```python
from build123d import *

# Parameters (mm, degrees)
SKETCH1_R               = 9.398
BOSS_EXTRUDE1_DEPTH     = 24.892
SKETCH2_R               = 2.54
CUT_EXTRUDE1_DEPTH      = 1
CUT_EXTRUDE1_DEPTH_BACK = 25.892
SKETCH3_R               = 3.9878
CUT_EXTRUDE2_DEPTH      = 12.446


with BuildPart() as part:
    # Sketch1 → Boss-Extrude1 (new body)
    with BuildSketch(Plane.XY):
        Circle(SKETCH1_R)
    extrude(amount=BOSS_EXTRUDE1_DEPTH)

    # Sketch2 → Cut-Extrude1 (cut, two sides)
    with BuildSketch(Plane(origin=(0, 0, 0), x_dir=(-1, 0, 0), z_dir=(0, 0, -1))) as cut_extrude1_sk:
        Circle(SKETCH2_R)
    extrude(amount=CUT_EXTRUDE1_DEPTH, mode=Mode.SUBTRACT)
    extrude(cut_extrude1_sk.sketch, amount=-CUT_EXTRUDE1_DEPTH_BACK, mode=Mode.SUBTRACT)

    # Sketch3 → Cut-Extrude2 (cut)
    with BuildSketch(Plane(origin=(0, 0, 0), x_dir=(-1, 0, 0), z_dir=(0, 0, -1))):
        Circle(SKETCH3_R)
    extrude(amount=-CUT_EXTRUDE2_DEPTH, mode=Mode.SUBTRACT)


solid = part.part
```
Check sheet for the modelled part. Datum: model origin and axes. Units: mm. A direction names the side the tool comes from. Coordinates: 2 decimals unless noted, no trailing zeros. Order: outer loops, then holes, each group sorted by start corner. A loop starts at its lowest first (then second) coordinate and runs counter-clockwise, first axis right, second up. Notation, with made-up numbers: M 22,52 L 70,52 A33 cw 70,81 Z; hole C 3,22 d11. An arc over 180 degrees is marked long. One line per question, with ' | ' between items. Start each with the question number.
Item 1: Sectioned sample at B-B on y = 1. Record the cut outline in (x, z), and give its area (3 significant figures).
Item 2: Sectioned sample at C-C on z = 17. Record the cut outline in (x, y).
Item 3: Gauge pin test, flat ends, axial feed: P1, Ø2, axis at y = -7.5, z = 16, coming from the +X side; P2, Ø5, axis at x = 0.5, y = -2, coming from the -Z side; P3, Ø8, axis at x = -5, z = 9.5, coming from the +Y side. Record the tip position at first contact, or that the pin passes through.
Item 4: Access from +Z, -Z, +X, -X, +Y, -Y to the whole of each face (thin tool, end or side, straight path). Record for faces 5 (the cylindrical face through (-3.804, 1.198, 6.136)), 6 (the flat face through (2, -2, 24.892)).
Item 5: Mould release check, pull along X, two halves, no side actions. Record for faces 1 (the cylindrical face through (0.33, 2.52, 18.58)), 2 (the flat face through (4, -2, 0)), 3 (the cylindrical face through (-1.22, 9.32, 12.27)), 4 (the flat face through (0, -3, 12.446)): pulls with the +X half, pulls with the -X half, needs draft (parallel to the pull), parting line crosses it, or undercut.
Item 6: Material ranges on line 1 (Y direction, x = 0, z = 9.5); line 2 (Z direction, x = 2, y = -2.75); line 3 (X direction, y = 1.5, z = 11.75), recorded low to high.
Item 7: Sectioned sample at D-D on x = 4.5. Record the cut outline in (y, z).
Item 8: Sectioned sample at A-A on x = 0. Record the cut outline in (y, z).
Answer below:
1) outline: M -9.34,0 L -3.86,0 L -3.86,12.45 L -2.33,12.45 L -2.33,24.89 L -9.34,24.89 Z; M 2.33,12.45 L 3.86,12.45 L 3.86,0 L 9.34,0 L 9.34,24.89 L 2.33,24.89 Z | area: 311 mm^2
2) outline: C 0,0 d18.8; hole C 0,0 d5.08
3) P1: stops at x = 6.79 | P2: stops at z = 0 | P3: stops at y = 9.34
4) face 5: -Z | face 6: +Z, +X, -X, +Y, -Y
5) face 1: undercut | face 2: needs draft | face 3: parting line crosses it | face 4: undercut
6) line 1: y = -9.4 to -3.99, 3.99 to 9.4 | line 2: z = 12.45 to 24.89 | line 3: x = -9.28 to -3.69, 3.69 to 9.28
7) outline: M -8.25,0 L 8.25,0 L 8.25,24.89 L -8.25,24.89 Z
8) outline: M -9.4,0 L -3.99,0 L -3.99,12.45 L -2.54,12.45 L -2.54,24.89 L -9.4,24.89 Z; M 2.54,12.45 L 3.99,12.45 L 3.99,0 L 9.4,0 L 9.4,24.89 L 2.54,24.89 Z
